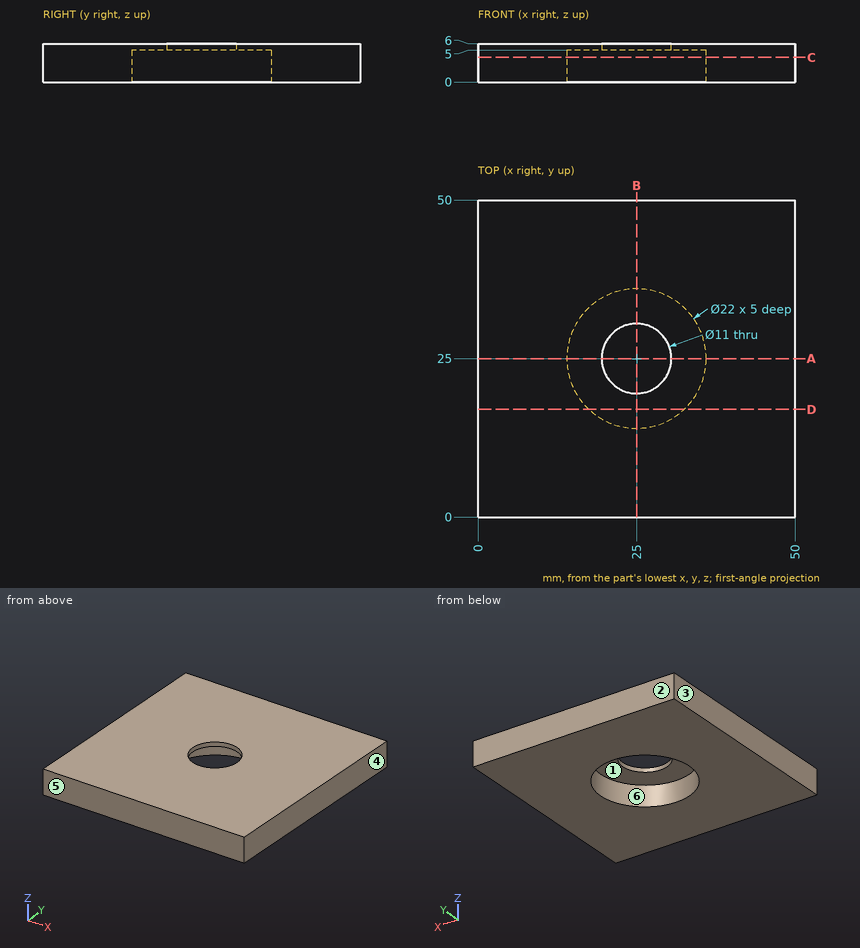
Print and shaded views of the part. All mm, measured from the part's lowest x, y and z. A direction names the side the tool comes from. Give positions to 0.01 mm unless a question says otherwise; leave off trailing zeros. Order: outer loops, then holes, each group sorted by start corner. A loop starts at its lowest first (then second) coordinate and runs counter-clockwise, first axis right, second up. Notation, with made-up numbers: (-17.75, -1.5) - (24.25, -1.5) arc R13 cw to (24.25, 13.5) - close; hole circle Ø3 at (53, 49.5). An arc over 180 degrees is marked (long way). One line per item, written item: value.
Item 1: Wall check: line 1 (Y direction, x = 25, z = 5.2); line 2 (Y direction, x = 25, z = 2.15); line 3 (Z direction, x = 33.5, y = 27.5). Give the ranges that are in metal, low to high.
Response values:
line 1: 0 to 19.5, 30.5 to 50
line 2: 0 to 14, 36 to 50
line 3: 5 to 6
Item 2: Tool access for the marked faces 1 and 2: list every direction of +Z, -Z, +X, -X, +Y, -Y with a clear straight run to the whole face (end or side of a thin tool).
Response values:
face 1: -Z
face 2: +Z, -Z, +X, -X, +Y
Item 3: Slice it at D-D (y = 17). List the corners of the cut face in (x, z), then the cut area to 3 significant figures.
Response values:
outline: (0, 0) - (17.45, 0) - (17.45, 5) - (32.55, 5) - (32.55, 0) - (50, 0) - (50, 6) - (0, 6) - close
area: 225 mm2
Item 4: Pin check, flat tip, straight feed: pin 1 Ø6.5 at (x, y) = (24.5, 20.5) entering from -Z. Stop position of the tip, or through.
Response values:
pin 1: z = 5
Item 5: Slice it at C-C (z = 3.9). List the corners of the cut face in (x, y).
Response values:
outline: (0, 0) - (50, 0) - (50, 50) - (0, 50) - close; hole circle Ø22 at (25, 25)
Item 6: Slice it at A-A (y = 25). List the corners of the cut face in (x, z), then the cut area to 3 significant figures.
Response values:
outline: (0, 0) - (14, 0) - (14, 5) - (19.5, 5) - (19.5, 6) - (0, 6) - close; (30.5, 5) - (36, 5) - (36, 0) - (50, 0) - (50, 6) - (30.5, 6) - close
area: 179 mm2
Item 7: Two-plate mould, pull along X, no slides. Class the marked faces 3, 4, 5 and 6: released by +X, released by -X, zero draft, split by the parting line, or undercut.
Response values:
face 3: released by -X
face 4: released by +X
face 5: zero draft
face 6: undercut
